Check sheet for the modelled part. Datum: model origin and axes. Units: mm. Round coordinates to 2 decimals unless told otherwise and drop trailing zeros. Write each loop counter-clockwise with the first axis right and the second up, starting at its lowest first coordinate (ties: lowest second). Pieces come first, ordered by that corner, then holes.
Item 1: Cross-section at A-A on x = -7.5. Enter the section's corners in (y, z).
Item 2: Cross-section at C-C on y = 3.3. Count the separate pieces of the cut face and the enclosed holes in it, plus the area to 3 significant figures.
Item 3: Go/stop test with a flat-tipped pin: pin 1 Ø2.5 at (x, z) = (-129.982, 24) entering from -Y. Record where the tip stops, or that it passes through.
Item 4: Cross-section at B-B on x = -62.5. Enter the section's corners in (y, z).
Item 5: Material ranges on line 1 (X direction, y = 0.5, z = 0); line 2 (Z direction, x = -55.5, y = 0.7); line 3 (X direction, y = 3.1, z = 5.5), recorded low to high.
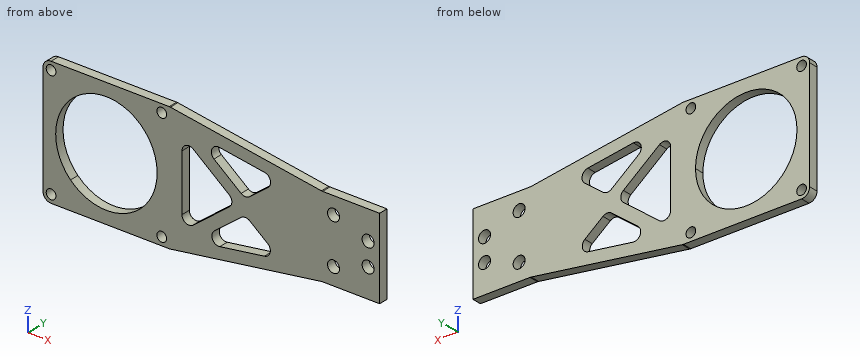
from build123d import *

# Parameters (mm, degrees)
SKETCH_1_W               = 25
SKETCH_1_H               = 35
SKETCH_1_R               = 2.6
EXTRUDE_1_DEPTH          = 4
EXTRUDE_2_DEPTH          = 4
FILLET_1_R               = 3.5
CUT_EXTRUDE_1_DEPTH      = 10
SKETCH_4_R               = 2.1
CUT_EXTRUDE_2_DEPTH      = 10
PATTERN_CIRCULAR_1_COUNT = 4
CUT_EXTRUDE_3_DEPTH      = 163


with BuildPart() as part:
    # 草图1 → 凸台-拉伸1 (new body)
    with BuildSketch(Plane(origin=(0, 0, 0), x_dir=(1, 0, 0), z_dir=(0, 1, 0))):
        Rectangle(SKETCH_1_W, SKETCH_1_H)
        with Locations(Location((7.5, 5, 0), (0, 0, 270))):
            Circle(SKETCH_1_R, mode=Mode.SUBTRACT)
        with Locations(Location((7.5, -5, 0), (0, 0, 270))):
            Circle(SKETCH_1_R, mode=Mode.SUBTRACT)
        with Locations(Location((-7.5, -10, 0), (0, 0, 270))):
            Circle(SKETCH_1_R, mode=Mode.SUBTRACT)
        with Locations(Location((-7.5, 10, 0), (0, 0, 270))):
            Circle(SKETCH_1_R, mode=Mode.SUBTRACT)
    extrude(amount=EXTRUDE_1_DEPTH)


with BuildPart() as body_2:
    # 草图2 → 凸台-拉伸2 (new body)
    with BuildSketch(Plane(origin=(0, 4, 0), x_dir=(1, 0, 0), z_dir=(0, 1, 0))):
        Polygon((-133.482, 27.5), (-78.482, 27.5), (-12.5, 17.5), (-12.5, -17.5), (-78.482, -27.5), (-133.482, -27.5), align=None)
    extrude(amount=-EXTRUDE_2_DEPTH)


with BuildPart() as part_1:
    add(part.part)

    # Combine 1: union body 2
    add(body_2.part)

    # 圆角1
    fillet_1_edges = [part_1.edges().sort_by_distance(p)[0] for p in [
        (-12.5, 2, -17.5),
        (-12.5, 2, 17.5),
        (-78.482, 2, 27.5),
        (-133.482, 2, 27.5),
        (-133.482, 2, -27.5),
        (-78.482, 2, -27.5),
    ]]
    fillet(fillet_1_edges, radius=FILLET_1_R)

    # 草图3 → 切除-拉伸1 (cut)
    with BuildSketch(Plane(origin=(0, 4, 0), x_dir=(1, 0, 0), z_dir=(0, 1, 0))):
        with BuildLine():
            ThreePointArc((-83.982, 0), (-97.562964488, 20.325349715), (-121.538349186, 15.556349186))
            Line((-121.538349186, 15.556349186), (-105.982, 0))
            Line((-105.982, 0), (-121.538349186, -15.556349186))
            ThreePointArc((-121.538349186, -15.556349186), (-97.562964488, -20.325349715), (-83.982, 0))
        make_face()
        with BuildLine():
            Line((-105.982, 0), (-121.538349186, 15.556349186))
            ThreePointArc((-121.538349186, 15.556349186), (-127.982, 0), (-121.538349186, -15.556349186))
            Line((-121.538349186, -15.556349186), (-105.982, 0))
        make_face()
    extrude(amount=-CUT_EXTRUDE_1_DEPTH, mode=Mode.SUBTRACT)

    # 草图4 → 切除-拉伸2 (cut)
    with BuildSketch(Plane(origin=(0, 4, 0), x_dir=(1, 0, 0), z_dir=(0, 1, 0))):
        with Locations(Location((-81.982, 24, 0), (0, 0, 270))):
            Circle(SKETCH_4_R)
    cut_extrude_2 = extrude(amount=-CUT_EXTRUDE_2_DEPTH, mode=Mode.SUBTRACT)

    # 阵列(圆周)1: 切除-拉伸2 ×4 about axis
    pattern_circular_1_axis = Axis((-105.982, 0, 0), (0, 1, 0))
    for i in range(1, PATTERN_CIRCULAR_1_COUNT):
        add(cut_extrude_2.rotate(pattern_circular_1_axis, i * 360 / PATTERN_CIRCULAR_1_COUNT), mode=Mode.SUBTRACT)

    # 草图5 → 切除-拉伸3 (cut)
    with BuildSketch(Plane(origin=(0, 82, 0), x_dir=(1, 0, 0), z_dir=(0, 1, 0))):
        with BuildLine():
            Line((-43.858652951, 4.717262465), (-36.024929121, 10.900937766))
            ThreePointArc((-36.024929121, 10.900937766), (-34.983693556, 14.023777786), (-37.434169796, 16.221837724))
            Line((-37.434169796, 16.221837724), (-56.789222754, 19.155221519))
            ThreePointArc((-56.789222754, 19.155221519), (-59.99021825, 17.384697858), (-59.100366311, 13.836558948))
            Line((-59.100366311, 13.836558948), (-47.579037182, 4.719499851))
            ThreePointArc((-47.579037182, 4.719499851), (-45.71923377, 4.072034614), (-43.858652951, 4.717262465))
        make_face()
        with BuildLine():
            Line((-35.914624614, -10.886886831), (-43.864253928, -4.59618552))
            ThreePointArc((-43.864253928, -4.59618552), (-45.72405734, -3.948720283), (-47.584638159, -4.593948133))
            Line((-47.584638159, -4.593948133), (-59.336609443, -13.870554782))
            ThreePointArc((-59.336609443, -13.870554782), (-60.230010812, -17.419276174), (-57.028296794, -19.191454741))
            Line((-57.028296794, -19.191454741), (-37.326696195, -16.205549403))
            ThreePointArc((-37.326696195, -16.205549403), (-34.876682386, -14.009233352), (-35.914624614, -10.886886831))
        make_face()
        with BuildLine():
            Line((-68.362482774, -14.625227843), (-52.732917259, -2.287780119))
            ThreePointArc((-52.732917259, -2.287780119), (-51.591694463, 0.065187331), (-52.730086351, 2.419525709))
            Line((-52.730086351, 2.419525709), (-68.359651866, 14.787514754))
            ThreePointArc((-68.359651866, 14.787514754), (-71.528006789, 15.135427044), (-73.221259435, 12.434980533))
            Line((-73.221259435, 12.434980533), (-73.221259435, -12.270456236))
            ThreePointArc((-73.221259435, -12.270456236), (-71.529630563, -14.970116398), (-68.362482774, -14.625227843))
        make_face()
    extrude(amount=-CUT_EXTRUDE_3_DEPTH, mode=Mode.SUBTRACT)


solid = part_1.part
Response values:
1. outline: (0, -17.5) - (4, -17.5) - (4, -12.6) - (0, -12.6) - close; (0, -7.4) - (4, -7.4) - (4, 7.4) - (0, 7.4) - close; (0, 12.6) - (4, 12.6) - (4, 17.5) - (0, 17.5) - close
2. separate pieces: 1
2. enclosed holes: 12
2. area: 4,320 mm2
3. pin 1: passes through
4. outline: (0, -25.08) - (4, -25.08) - (4, -10.15) - (0, -10.15) - close; (0, 10) - (4, 10) - (4, 25.08) - (0, 25.08) - close
5. line 1: x = -133.48 to -127.98, -83.98 to -73.22, -51.59 to 12.5
5. line 2: z = -24.02 to -18.96, -10.99 to -4.61, 4.47 to 10.84, 18.96 to 24.02
5. line 3: x = -133.48 to -127.28, -84.68 to -73.22, -56.8 to -48.73, -42.72 to 4.95, 10.05 to 12.5
